Can you work these out from the model? Positions are in its coordinate system, mm. A direction names the side the tool comes from. Coordinates: 2 decimals unless noted, no trailing zeros. Order: outer loops, then holes, each group sorted by start corner. A loop starts at its lowest first (then second) coordinate and runs counter-clockwise, first axis right, second up. Notation, with made-up numbers: (77.5, 27.5) -> (81.5, 27.5) arc R10 ccw to (81.5, 42.5) -> close; hole circle Ø5 at (-9.5, -28.5). An arc over 180 degrees is marked (long way). Answer as a JSON object with one key per item and string values. Group by question number.
(1) I need wall thicknesses on line 1 (Z direction, x = -46, y = -4.5); line 2 (X direction, y = -5.25, z = -0.5); line 3 (X direction, y = -1, z = -12). Which ranges of each line are inside material? Lowest first, please.
(2) I want a section at D-D, the plane x = -33.5. List the corners of the cut face in (y, z) for me, plus the area to 3 significant figures.
(3) For pin 1 (2.5 mm diameter, centred on x = -45, y = -3.5, fed in from +Z); pin 2 (3 mm diameter, centred on y = -4.5, z = 3, fed in from -X); pin 3 (3 mm diameter, centred on y = -3.5, z = 34, fed in from -X), each with a flat end and sliding along its axis, tell me the tip position at first contact or that it passes through.
(4) I want a section at B-B, the plane z = -7. List the corners of the cut face in (x, y) for me, plus the area to 3 significant figures.
(5) I want a section at C-C, the plane z = -28.5. List the corners of the cut face in (x, y) for me, plus the area to 3 significant figures.
(6) Which directions (+Z, -Z, +X, -X, +Y, -Y) give clear straight access to the entire face, cutting with the end or side of a thin tool? Please do faces 1 (the flat face through (-51, -3, -20.447)), 2 (the flat face through (-54, -3, 22.86)), 3 (the flat face through (-46.203, -3, -22)).
(7) If we mould it in two halves opening along X, with no side actions, what happens to faces 4 (the flat face through (38.1, -3, 1)), 5 (the cylindrical face through (16.34, -3.13, -9.01)), 6 (the flat face through (-48, -3, -10.16)), 7 (the flat face through (-45, -3, -20.447))? For each: pulls with the +X half, pulls with the -X half, needs draft (parallel to the pull), parting line crosses it, or undercut.
(8) I want a section at A-A, the plane x = 2.5. List the corners of the cut face in (y, z) for me, plus the area to 3 significant figures.
from build123d import *

# Parameters (mm, degrees)
BOSS_EXTRUDE1_DEPTH = 6.35


with BuildPart() as part:
    # Sketch1 → Boss-Extrude1 (new body)
    with BuildSketch(Plane(origin=(0, 0, 0), x_dir=(1, 0, 0), z_dir=(0, 1, 0))):
        Polygon((-25.4, -38.1), (38.1, -38.1), (38.1, 38.1), (-25.4, 38.1), (-25.4, 22.86), (-38.1, 22.86), (-46.2026, 22.86), (-46.2026, 20.447), (-44.0944, 20.447), (-44.0944, 17.78), (-51.9684, 17.78), (-51.9684, 20.447), (-49.8602, 20.447), (-49.8602, 22.86), (-57.9628, 22.86), (-57.9628, 10.16), (-38.1, 10.16), (-38.1, -10.16), (-57.9628, -10.16), (-57.9628, -22.86), (-49.8602, -22.86), (-49.8602, -20.447), (-51.9684, -20.447), (-51.9684, -17.78), (-44.0944, -17.78), (-44.0944, -20.447), (-46.2026, -20.447), (-46.2026, -22.86), (-38.1, -22.86), (-25.4, -22.86), align=None)
        with BuildLine():
            Line((7.227071664, -18.99759929), (12.838867764, -15.757627301))
            Line((12.838867764, -15.757627301), (11.99371709, -14.293783392))
            ThreePointArc((11.99371709, -14.293783392), (16.159242555, 9.329543039), (-6.381920989, 17.533755382))
            Line((-6.381920989, 17.533755382), (-7.227071664, 18.99759929))
            Line((-7.227071664, 18.99759929), (-12.838867764, 15.757627301))
            Line((-12.838867764, 15.757627301), (-11.99371709, 14.293783392))
            ThreePointArc((-11.99371709, 14.293783392), (-16.159242555, -9.329543039), (6.381920989, -17.533755382))
            Line((6.381920989, -17.533755382), (7.227071664, -18.99759929))
        make_face(mode=Mode.SUBTRACT)
    extrude(amount=-BOSS_EXTRUDE1_DEPTH)


solid = part.part
Computed values:
{
 "1": {"line 1": "z = -22.86 to -20.45, -17.78 to -10.16, 10.16 to 17.78, 20.45 to 22.86", "line 2": "x = -38.1 to -18.65, 18.65 to 38.1", "line 3": "x = -57.96 to -14.29, 14.29 to 38.1"},
 "2": {"outline": "(-6.35, -22.86) -> (0, -22.86) -> (0, 22.86) -> (-6.35, 22.86) -> close", "area": "290 mm2"},
 "3": {"pin 1": "stops at z = 22.86", "pin 2": "stops at x = -38.1", "pin 3": "stops at x = -25.4"},
 "4": {"outline": "(-38.1, -6.35) -> (-17.3, -6.35) -> (-17.3, 0) -> (-38.1, 0) -> close; (17.3, -6.35) -> (38.1, -6.35) -> (38.1, 0) -> (17.3, 0) -> close", "area": "264 mm2"},
 "5": {"outline": "(-25.4, -6.35) -> (38.1, -6.35) -> (38.1, 0) -> (-25.4, 0) -> close", "area": "403 mm2"},
 "6": {"face 1": "+Y, -Y", "face 2": "+Z, -X, +Y, -Y", "face 3": "-Z, +Y, -Y"},
 "7": {"face 4": "pulls with the +X half", "face 5": "undercut", "face 6": "needs draft", "face 7": "undercut"},
 "8": {"outline": "(-6.35, -38.1) -> (0, -38.1) -> (0, -18.49) -> (-6.35, -18.49) -> close; (-6.35, 18.49) -> (0, 18.49) -> (0, 38.1) -> (-6.35, 38.1) -> close", "area": "249 mm2"}
}
